from build123d import *

# Parameters (mm, degrees)
SKETCH1_R           = 20
SKETCH1_R_2         = 9
BOSS_EXTRUDE3_DEPTH = 21
BOSS_EXTRUDE4_DEPTH = 16
BOSS_EXTRUDE5_START = -16
SKETCH2_R           = 30
SKETCH2_R_2         = 15
BOSS_EXTRUDE5_DEPTH = 25
BOSS_EXTRUDE6_DEPTH = 16
SKETCH4_R           = 20
SKETCH4_R_2         = 8
BOSS_EXTRUDE7_DEPTH = 12
BOSS_EXTRUDE9_DEPTH = 6


with BuildPart() as part:
    # Sketch1 → Boss-Extrude3 (new body)
    with BuildSketch(Plane(origin=(0, 0, 0), x_dir=(1, 0, 0), z_dir=(0, 1, 0))):
        with Locations(Location((0, 0, 0), (0, 0, 90))):
            Circle(SKETCH1_R)
        with Locations(Location((0, 0, 0), (0, 0, 90))):
            Circle(SKETCH1_R_2, mode=Mode.SUBTRACT)
    extrude(amount=BOSS_EXTRUDE3_DEPTH)

    # Sketch1_5 → Boss-Extrude4 (add)
    with BuildSketch(Plane(origin=(0, 0, 0), x_dir=(1, 0, 0), z_dir=(0, 1, 0))):
        with BuildLine():
            ThreePointArc((-6.177666108, 19.021998882), (11.756842217, 16.179513623), (20, 0))
            Line((20, 0), (120, 0))
            Line((120, 0), (120, 60))
            Line((120, 60), (-6.177666108, 19.021998882))
        make_face()
        with BuildLine():
            Line((120, 0), (20, 0))
            ThreePointArc((20, 0), (11.756842217, -16.179513623), (-6.177666108, -19.021998882))
            Line((-6.177666108, -19.021998882), (120, -60))
            Line((120, -60), (120, 0))
        make_face()
        Polygon((136, -60), (136, 60), (120, 60), (120, 0), (120, -60), align=None)
    extrude(amount=BOSS_EXTRUDE4_DEPTH)



with BuildPart() as body_2:
    # Sketch2 → Boss-Extrude5 (new body)
    with BuildSketch(Plane(origin=(136, 0, 0), x_dir=(0, 0, -1), z_dir=(1, 0, 0)).offset(BOSS_EXTRUDE5_START)):
        with Locations((0, 106)):
            Circle(SKETCH2_R)
        with Locations((0, 106)):
            Circle(SKETCH2_R_2, mode=Mode.SUBTRACT)
    extrude(amount=BOSS_EXTRUDE5_DEPTH)


with BuildPart() as part_1:
    add(part.part)

    add(body_2.part)  # Boss-Extrude6 merges body 2
    # Sketch2_4 → Boss-Extrude6 (add)
    with BuildSketch(Plane(origin=(136, 0, 0), x_dir=(0, 0, -1), z_dir=(1, 0, 0))):
        with BuildLine():
            Line((-28.597626566, 115.065084378), (-60, 16))
            Line((-60, 16), (60, 16))
            Line((60, 16), (28.597626566, 115.065084378))
            ThreePointArc((28.597626566, 115.065084378), (29.64733375, 110.586458493), (30, 106))
            ThreePointArc((30, 106), (-4.586458493, 76.35266625), (-28.597626566, 115.065084378))
        make_face()
    extrude(amount=-BOSS_EXTRUDE6_DEPTH)



with BuildPart() as body_2_2:
    # Sketch4 → Boss-Extrude7 (new, symmetric)
    with BuildSketch(Plane.XY):
        with Locations((70, 61)):
            Circle(SKETCH4_R)
        with Locations((70, 61)):
            Circle(SKETCH4_R_2, mode=Mode.SUBTRACT)
    extrude(amount=BOSS_EXTRUDE7_DEPTH, both=True)


with BuildPart() as part_2:
    add(part_1.part)

    add(body_2_2.part)  # Boss-Extrude9 merges body 2 2
    # Sketch4_4 → Boss-Extrude9 (add, symmetric)
    with BuildSketch(Plane.XY):
        with BuildLine():
            Line((120, 81), (70, 81))
            ThreePointArc((70, 81), (84.142135624, 75.142135624), (90, 61))
            ThreePointArc((90, 61), (64.033186243, 41.910811081), (53.560286641, 72.390163506))
            Line((53.560286641, 72.390163506), (17.954899118, 21))
            Line((17.954899118, 21), (17.954899118, 16))
            Line((17.954899118, 16), (20, 16))
            Line((20, 16), (120, 16))
            Line((120, 16), (120, 81))
        make_face()
    extrude(amount=BOSS_EXTRUDE9_DEPTH, both=True)


solid = part_2.part
Work out the finished part from the listing and answer in its coordinate system (mm). A direction names the side the tool comes from. Give positions to 0.01 mm unless a question says otherwise; leave off trailing zeros. Order: outer loops, then holes, each group sorted by start corner. A loop starts at its lowest first (then second) coordinate and runs counter-clockwise, first axis right, second up. Notation, with made-up numbers: (-25, 67) - (18, 67) arc R28 ccw to (18, 86) - close; hole circle Ø4 at (-17, 75.25). An arc over 180 degrees is marked (long way). Answer as CSV lines item,"result". Start each with the question number.
Q1. The part is cut by section C-C (x = -3.5). Write down the section's boundary in (y, z), then the cut area to 3 significant figures.
Q2. The part is cut by section D-D (y = 106). Write down the section's boundary in (x, z), then the cut area to 3 significant figures.
Q3. For faces 1 (the face through (80, 42, -6)), 2 (the face through (67.4, 80.83, 0.17)), 3 (the face through (80, 42, 6)), 4 (the face through (70, 52, 12)), 5 (the face through (-19.984, 12.686, -0.794)), determine the directions among +Z, -Z, +X, -X, +Y, -Y from which every point of the face is accessible in a straight line to the end or side of a thin tool.
Q4. Given pin 1 Ø21 at (x, y) = (70, 61) entering from -Z; pin 2 Ø16 at (x, z) = (0, 0) entering from +Y; pin 3 Ø6 at (x, y) = (65.5, 46.5) entering from +Z; pin 4 Ø4 at (x, y) = (106, 50) entering from +Z, each flat-ended and moving along its own axis, determine where each tip first touches the part or whether it passes through.
Q5. The part is cut by section B-B (y = 10). Write down the section's boundary in (x, z).
Q6. The part is cut by section A-A (z = 0). Write down the section's boundary in (x, y), then the cut area to 3 significant figures.
Q7. The mould has two halves that part along X. Classify faces 6 (the face through (68.959, 68.932, -0.168)), 7 (the face through (128.112, 66.226, 44.079)), 8 (the face through (145, 120, -6)): +X half, -X half, draft (parallel to the pull), parting line (faces both ways), or undercut.
Q8. Find the intervals of material crossed by L1, parallel to Y at x = 70, z = -4; L2, parallel to Y at x = 128, z = 0; L3, parallel to Z at x = 82, y = 41, in increasing order. Write a range as [from, to].
Check result:
1,outline,"(0, -19.89) - (16, -19.89) - (16, -19.69) - (21, -19.69) - (21, -8.29) - (0, -8.29) - close; (0, 8.29) - (21, 8.29) - (21, 19.69) - (16, 19.69) - (16, 19.89) - (0, 19.89) - close"
1,area,"485 mm²"
2,outline,"(120, -31.47) - (136, -31.47) - (136, -30) - (145, -30) - (145, -15) - (120, -15) - close; (120, 15) - (145, 15) - (145, 30) - (136, 30) - (136, 31.47) - (120, 31.47) - close"
2,area,"797 mm²"
3,face 1,"-Z"
3,face 2,"none"
3,face 3,"+Z"
3,face 4,"+Z, -X, +Y"
3,face 5,"+Y"
4,pin 1,"stops at z = -12"
4,pin 2,"passes through"
4,pin 3,"stops at z = 12"
4,pin 4,"stops at z = 6"
5,outline,"(-6.18, -19.02) - (120, -60) - (136, -60) - (136, 60) - (120, 60) - (-6.18, 19.02) arc R20 ccw to start; hole circle Ø18 at (0, 0)"
6,outline,"(-20, 0) - (-9, 0) - (-9, 21) - (-20, 21) - close; (9, 0) - (136, 0) - (136, 76) - (145, 76) - (145, 91) - (120, 91) - (120, 81) - (70, 81) arc R20 ccw to (53.56, 72.39) - (17.95, 21) - (9, 21) - close; (120, 121) - (145, 121) - (145, 136) - (120, 136) - close; hole circle Ø16 at (70, 61)"
6,area,"9,190 mm²"
7,face 6,"undercut"
7,face 7,"draft"
7,face 8,"+X half"
8,L1,"y = [0, 53], [69, 81]"
8,L2,"y = [0, 91], [121, 136]"
8,L3,"z = [-6, 6]"
